Could you check a few things on this model? Use its own coordinates, in mm. Give positions to 0.01 mm unless a question says otherwise; leave off trailing zeros. Order: outer loops, then holes, each group sorted by start corner. A loop starts at its lowest first (then second) coordinate and runs counter-clockwise, first axis right, second up. Notation, with made-up numbers: (56, -25.75) -> (69, -25.75) arc R28 cw to (69, 4.25) -> close; hole circle Ø11 at (58, 86). An arc over 180 degrees is marked (long way). One line per item, written item: value.
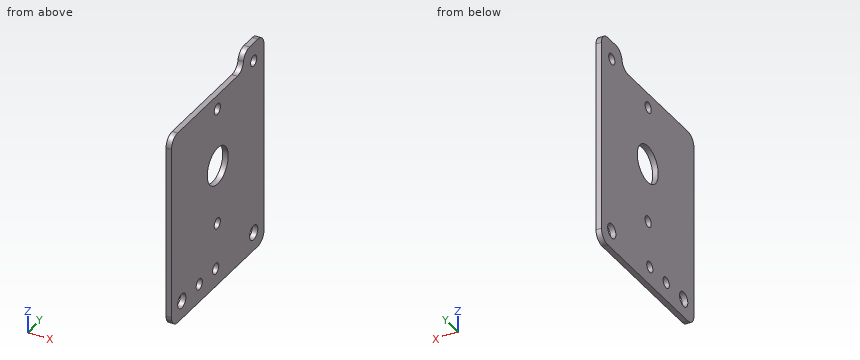
```python
from build123d import *

# Parameters (mm, degrees)
SKETCH_1_W          = 53.5
SKETCH_1_H          = 45
SKETCH_1_R          = 5.1
SKETCH_1_R_2        = 2
SKETCH_1_R_3        = 1.5
EXTRUDE_1_DEPTH     = 1.5
SKETCH_3_W          = 5
SKETCH_3_H          = 10
EXTRUDE_2_DEPTH     = 1.5
SKETCH_4_R          = 1.5
CUT_EXTRUDE_2_DEPTH = 39.943067419
FILLET_1_R          = 3
FILLET_2_R          = 3


with BuildPart() as part:
    # ｽｹｯﾁ1 → ﾎﾞｽ - 押し出し1 (new body)
    with BuildSketch(Plane(origin=(0, 0, 0), x_dir=(0, 0, -1), z_dir=(1, 0, 0))):
        Rectangle(SKETCH_1_W, SKETCH_1_H)
        with Locations((-6.75, 0)):
            Circle(SKETCH_1_R, mode=Mode.SUBTRACT)
        with Locations((21.75, 17.5)):
            Circle(SKETCH_1_R_2, mode=Mode.SUBTRACT)
        with Locations((-22.88, -0.21)):
            Circle(SKETCH_1_R_3, mode=Mode.SUBTRACT)
        with Locations(Location((9.38, -0.21, 0), (0, 0, 180))):
            Circle(SKETCH_1_R_3, mode=Mode.SUBTRACT)
        with Locations((21.75, -1)):
            Circle(SKETCH_1_R_3, mode=Mode.SUBTRACT)
        with Locations(Location((21.75, -17.5, 0), (0, 0, 180))):
            Circle(SKETCH_1_R_2, mode=Mode.SUBTRACT)
        with Locations((21.75, -9)):
            Circle(SKETCH_1_R_3, mode=Mode.SUBTRACT)
    extrude(amount=EXTRUDE_1_DEPTH)

    # ｽｹｯﾁ3 → ﾎﾞｽ - 押し出し2 (add)
    with BuildSketch(Plane(origin=(1.5, 0, 0), x_dir=(0, 0, -1), z_dir=(1, 0, 0))):
        with Locations((-29.25, 17.5)):
            Rectangle(SKETCH_3_W, SKETCH_3_H)
    extrude(amount=-EXTRUDE_2_DEPTH)

    # ｽｹｯﾁ4 → ｶｯﾄ - 押し出し2 (cut, through all)
    with BuildSketch(Plane(origin=(1.5, 0, 0), x_dir=(0, 0, -1), z_dir=(1, 0, 0))):
        with Locations((-26.75, 17.5)):
            Circle(SKETCH_4_R)
    extrude(amount=-CUT_EXTRUDE_2_DEPTH, mode=Mode.SUBTRACT)

    # ﾌｨﾚｯﾄ1
    fillet_1_edges = [part.edges().sort_by_distance(p)[0] for p in [
        (0.75, 22.5, 31.75),
        (0.75, 12.5, 31.75),
        (0.75, -22.5, -26.75),
        (0.75, -22.5, 26.75),
        (0.75, 22.5, -26.75),
    ]]
    fillet(fillet_1_edges, radius=FILLET_1_R)

    # ﾌｨﾚｯﾄ2
    fillet_2_edges = [part.edges().sort_by_distance(p)[0] for p in [
        (0.75, 12.5, 26.75),
    ]]
    fillet(fillet_2_edges, radius=FILLET_2_R)


solid = part.part
```
1) Suppose I cut it at A-A, the plane z = -9.38. Write out the boundary of the cut face in (x, y), then the cut area to 3 significant figures.
Answer below:
outline: (0, -22.5) -> (1.5, -22.5) -> (1.5, -1.71) -> (0, -1.71) -> close; (0, 1.29) -> (1.5, 1.29) -> (1.5, 22.5) -> (0, 22.5) -> close
area: 63.0 mm2
2) For P1, Ø1.5, axis at y = -4, z = 2.5, coming from the -X side, with a flat end and sliding along its axis, tell me the tip position at first contact or that it passes through.
Answer below:
P1: stops at x = 0
3) Suppose I cut it at D-D, the plane z = 6. Write out the boundary of the cut face in (x, y).
Answer below:
outline: (0, -22.5) -> (1.5, -22.5) -> (1.5, -5.04) -> (0, -5.04) -> close; (0, 5.04) -> (1.5, 5.04) -> (1.5, 22.5) -> (0, 22.5) -> close
4) Suppose I cut it at B-B, the plane z = -21.75. Write out the boundary of the cut face in (x, y).
Answer below:
outline: (0, -22.5) -> (1.5, -22.5) -> (1.5, -19.5) -> (0, -19.5) -> close; (0, -15.5) -> (1.5, -15.5) -> (1.5, -10.5) -> (0, -10.5) -> close; (0, -7.5) -> (1.5, -7.5) -> (1.5, -2.5) -> (0, -2.5) -> close; (0, 0.5) -> (1.5, 0.5) -> (1.5, 15.5) -> (0, 15.5) -> close; (0, 19.5) -> (1.5, 19.5) -> (1.5, 22.5) -> (0, 22.5) -> close
5) Suppose I cut it at C-C, the plane x = 0.9. State how many separate pieces and enclosed holes the cut face has, then the cut area to 3 significant figures.
Answer below:
separate pieces: 1
enclosed holes: 8
area: 2,310 mm2
6) If I drill on line 1 along Y through (x, z) = (0.2, -23.5); line 2 along Y through (x, z) = (0.2, -23); line 3 along Y through (x, z) = (1.1, 6.75), over which ranges is the centre line in solid material (lowest first)?
Answer below:
line 1: y = -22.5 to -18.47, -16.53 to 16.53, 18.47 to 22.5
line 2: y = -22.5 to -19.06, -15.94 to -9.83, -8.17 to -1.83, -0.17 to 15.94, 19.06 to 22.5
line 3: y = -22.5 to -5.1, 5.1 to 22.5
